```python
from build123d import *

# Parameters (mm, degrees)
SKETCH_1_W          = 30
SKETCH_1_H          = 15
EXTRUDE_1_DEPTH     = 2
FILLET_1_R          = 7.5
SKETCH_2_R          = 2
CUT_EXTRUDE_1_DEPTH = 2


with BuildPart() as part:
    # 草图1 → 凸台-拉伸1 (new body)
    with BuildSketch(Plane.XY):
        Rectangle(SKETCH_1_W, SKETCH_1_H)
    extrude(amount=EXTRUDE_1_DEPTH)

    # 圆角1
    fillet_1_edges = [part.edges().sort_by_distance(p)[0] for p in [
        (15, -7.5, 1),
        (-15, -7.5, 1),
        (-15, 7.5, 1),
        (15, 7.5, 1),
    ]]
    fillet(fillet_1_edges, radius=FILLET_1_R - 0.0001)  # a hair under: the kernel refuses the full size

    # 草图2 → 切除-拉伸1 (cut)
    with BuildSketch(Plane.XY.offset(2)):
        with Locations((7.5, 0)):
            Circle(SKETCH_2_R)
        with Locations(Location((-7.5, 0, 0), (0, 0, 180))):
            Circle(SKETCH_2_R)
    extrude(amount=-CUT_EXTRUDE_1_DEPTH, mode=Mode.SUBTRACT)


solid = part.part
```
Build history of the part. All positions in model axes, mm. Give positions to 0.01 mm unless a question says otherwise; leave off trailing zeros. Loops run counter-clockwise (first coordinate to the right, second up) from the corner with the lowest first, then second, coordinate; pieces in that order, holes last.
Item 1: Drill centre lines: line 1 (Y direction, x = 7.5, z = 1.1); line 2 (X direction, y = -0.75, z = 0.9); line 3 (X direction, y = -1, z = 0.95). Where is each one in solid material? Low to high.
Answers follow:
line 1: y = -7.5 to -2, 2 to 7.5
line 2: x = -14.96 to -9.35, -5.65 to 5.65, 9.35 to 14.96
line 3: x = -14.93 to -9.23, -5.77 to 5.77, 9.23 to 14.93
Item 2: Pull direction Y, two halves, no side cores. Call faces 1 (the face through (0, 0, 0)), 2 (the face through (-5.502, -0.088, 1.014)), 3 (the face through (12.861, 5.245, 1.014)), 4 (the face through (5.502, 0.088, 1.014)): released by +Y, released by -Y, zero draft, split by the parting line, or undercut.
Answers follow:
face 1: zero draft
face 2: undercut
face 3: released by +Y
face 4: undercut
Item 3: Slice it at B-B, the plane x = 11. List the corners of the cut face in (y, z), and give its area (3 significant figures).
Answers follow:
outline: (-6.63, 0) - (6.63, 0) - (6.63, 2) - (-6.63, 2) - close
area: 26.5 mm2
Item 4: Flat gauge pins, fed straight in: pin 1 (5 mm diameter, centred on x = -7.5, y = 0, fed in from -Z); pin 2 (3 mm diameter, centred on x = 7.5, y = 0, fed in from +Z). Where does each tip first touch, or does it go through?
Answers follow:
pin 1: stops at z = 0
pin 2: passes through
Item 5: Slice it at A-A, the plane z = 0.9. Give the number of separate pieces and of enclosed holes in the cut face, and give its area (3 significant figures).
Answers follow:
separate pieces: 1
enclosed holes: 2
area: 377 mm2
Item 6: Slice it at C-C, the plane y = 3. List the corners of the cut face in (x, z).
Answers follow:
outline: (-14.37, 0) - (14.37, 0) - (14.37, 2) - (-14.37, 2) - close
